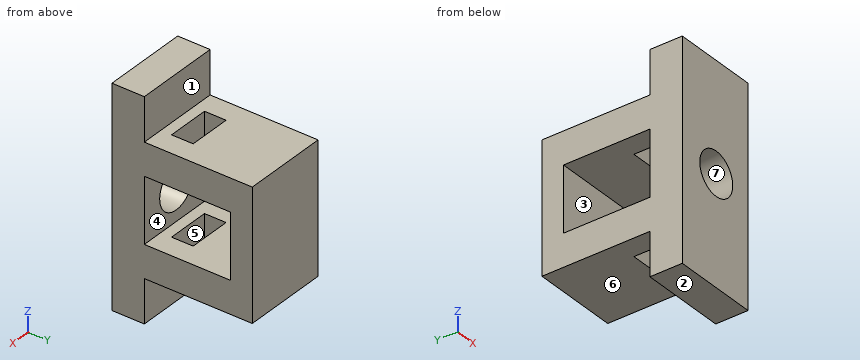
from build123d import *

# Parameters (mm, degrees)
SKETCH1_W           = 30
SKETCH1_H           = 40
BOSS_EXTRUDE1_DEPTH = 40
SKETCH2_W           = 20
SKETCH2_H           = 10
CUT_EXTRUDE1_DEPTH  = 107.082782983
SKETCH3_R           = 10
CUT_EXTRUDE2_DEPTH  = 109.757771635


with BuildPart() as part:
    # Sketch1 → Boss-Extrude1 (new body)
    with BuildSketch(Plane(origin=(0, 0, 0), x_dir=(0, 0, -1), z_dir=(1, 0, 0))):
        Polygon((-12.089517741, -57.039958323), (-12.089517741, -42.039958323), (7.910482259, -42.039958323), (7.910482259, 7.960041677), (67.910482259, 7.960041677), (67.910482259, -42.039958323), (87.910482259, -42.039958323), (87.910482259, -57.039958323), align=None)
        with Locations((37.910482259, -22.039958323)):
            Rectangle(SKETCH1_W, SKETCH1_H, mode=Mode.SUBTRACT)
    extrude(amount=BOSS_EXTRUDE1_DEPTH)

    # Sketch2 → Cut-Extrude1 (cut, through all)
    with BuildSketch(Plane.XY.offset(-7.910482259)):
        with Locations((20, -32.039958323)):
            Rectangle(SKETCH2_W, SKETCH2_H)
    extrude(amount=-CUT_EXTRUDE1_DEPTH, mode=Mode.SUBTRACT)

    # Sketch3 → Cut-Extrude2 (cut, through all)
    with BuildSketch(Plane(origin=(0, -42.039958323, 0), x_dir=(1, 0, 0), z_dir=(0, 1, 0))):
        with Locations(Location((20.652222237, 37.801778553, 0), (0, 0, 270))):
            Circle(SKETCH3_R)
    extrude(amount=-CUT_EXTRUDE2_DEPTH, mode=Mode.SUBTRACT)


solid = part.part
Can you work these out from the model? Positions are in its coordinate system, mm. Face numbers are marked on the shaded views. A direction names the side the tool comes from. Round coordinates to 2 decimals unless told otherwise and drop trailing zeros. Loops run counter-clockwise (first coordinate to the right, second up) from the corner with the lowest first, then second, coordinate; pieces in that order, holes last. Notation, with made-up numbers: (-28.75, 77.5) - (-24.75, 77.5) arc R23 cw to (-24.75, 91.5) - close; hole circle Ø5 at (58, -36). An arc over 180 degrees is marked (long way). Answer in a Markdown table with one row per item. Add a question column.
Q1. I want a section at D-D on y = -31. List the corners of the cut face in (x, z) for me, and give its area (3 significant figures).
Q2. Which directions (+Z, -Z, +X, -X, +Y, -Y) give clear straight access to the entire face, cutting with the end or side of a thin tool? Please do the marked faces 4, 5, 6 and 7.
Q3. I want a section at A-A on y = -4. List the corners of the cut face in (x, z) for me, and give its area (3 significant figures).
Q4. For pin 1 Ø12 at (x, y) = (26, -16.5) entering from -Z; pin 2 Ø5 at (x, y) = (10, -41) entering from -Z; pin 3 Ø16 at (x, z) = (23, 2.5) entering from +Y; pin 4 Ø12 at (x, y) = (28.5, -20.5) entering from +Z, each with a flat end and sliding along its axis, tell me the tip position at first contact or that it passes through.
Q5. I want a section at C-C on x = 6. List the corners of the cut face in (y, z) for me.
Q6. We'd pull the mould along Y, two halves only. Please class the marked faces 1, 2 and 3: pulls with the +Y half, pulls with the -Y half, needs draft (parallel to the pull), parting line crosses it, or undercut.
Q7. I want a section at B-B on z = -64. List the corners of the cut face in (x, y) for me.
Q8. I need wall thicknesses on L1, parallel to Y at x = 7.5, z = -26; L2, parallel to Z at x = 31, y = -16; L3, parallel to Y at x = 24, z = -67. Which ranges of each line are inside material? Lowest first, please.
A:
| question | item | result |
|---|---|---|
| 1 | outline | (0, -67.91) - (10, -67.91) - (10, -52.91) - (0, -52.91) - close; (0, -22.91) - (10, -22.91) - (10, -7.91) - (0, -7.91) - close; (30, -67.91) - (40, -67.91) - (40, -52.91) - (30, -52.91) - close; (30, -22.91) - (40, -22.91) - (40, -7.91) - (30, -7.91) - close |
| 1 | area | 600 mm^2 |
| 2 | face 4 | +X, -X |
| 2 | face 5 | +Z, -Z |
| 2 | face 6 | -Z, +X, -X, +Y |
| 2 | face 7 | -Y |
| 3 | outline | (0, -67.91) - (40, -67.91) - (40, -52.91) - (0, -52.91) - close; (0, -22.91) - (40, -22.91) - (40, -7.91) - (0, -7.91) - close |
| 3 | area | 1,200 mm^2 |
| 4 | pin 1 | z = -67.91 |
| 4 | pin 2 | z = -87.91 |
| 4 | pin 3 | y = -42.04 |
| 4 | pin 4 | z = -7.91 |
| 5 | outline | (-57.04, -87.91) - (-42.04, -87.91) - (-42.04, -67.91) - (7.96, -67.91) - (7.96, -7.91) - (-42.04, -7.91) - (-42.04, 12.09) - (-57.04, 12.09) - close; hole (-42.04, -52.91) - (-2.04, -52.91) - (-2.04, -22.91) - (-42.04, -22.91) - close |
| 6 | face 1 | pulls with the +Y half |
| 6 | face 2 | needs draft |
| 6 | face 3 | undercut |
| 7 | outline | (0, -57.04) - (40, -57.04) - (40, 7.96) - (0, 7.96) - close; hole (10, -37.04) - (30, -37.04) - (30, -27.04) - (10, -27.04) - close |
| 8 | L1 | -57.04 to -42.04, -2.04 to 7.96 |
| 8 | L2 | -67.91 to -52.91, -22.91 to -7.91 |
| 8 | L3 | -57.04 to -37.04, -27.04 to 7.96 |
